```python
from build123d import *

# Parameters (mm, degrees)
SKETCH1_W           = 50.8
SKETCH1_H           = 38.1
SKETCH1_R           = 2.38125
BOSS_EXTRUDE1_DEPTH = 25.4
CUT_EXTRUDE1_DEPTH  = 58.410261207
FILLET1_R           = 6.35
SKETCH3_R           = 2.921
CUT_EXTRUDE2_DEPTH  = 25.4


with BuildPart() as part:
    # Sketch1 → Boss-Extrude1 (new body)
    with BuildSketch(Plane(origin=(0, 0, 0), x_dir=(1, 0, 0), z_dir=(0, 1, 0))):
        with Locations((-9.229006509, -1.483233189)):
            Rectangle(SKETCH1_W, SKETCH1_H)
        with Locations(Location((-28.279006509, 7.406766811, 0), (0, 0, 270))):
            Circle(SKETCH1_R, mode=Mode.SUBTRACT)
        with Locations(Location((-28.279006509, -1.483233189, 0), (0, 0, 270))):
            Circle(SKETCH1_R, mode=Mode.SUBTRACT)
        with Locations(Location((-28.279006509, -10.373233189, 0), (0, 0, 270))):
            Circle(SKETCH1_R, mode=Mode.SUBTRACT)
        with Locations(Location((9.820993491, -10.373233189, 0), (0, 0, 270))):
            Circle(SKETCH1_R, mode=Mode.SUBTRACT)
        with Locations(Location((9.820993491, -1.483233189, 0), (0, 0, 270))):
            Circle(SKETCH1_R, mode=Mode.SUBTRACT)
        with Locations(Location((9.820993491, 7.406766811, 0), (0, 0, 270))):
            Circle(SKETCH1_R, mode=Mode.SUBTRACT)
    extrude(amount=BOSS_EXTRUDE1_DEPTH)

    # Sketch2 → Cut-Extrude1 (cut, through all)
    with BuildSketch(Plane.XY.offset(20.533233189)):
        with BuildLine():
            Line((-21.929006509, 0), (3.470993491, 0))
            ThreePointArc((3.470993491, 0), (-9.229006509, 12.7), (-21.929006509, 0))
        make_face()
        Polygon((-25.739006509, 25.4), (7.280993491, 25.4), (16.170993491, 25.4), (16.170993491, 6.35), (3.470993491, 6.35), (3.470993491, 19.05), (-21.929006509, 19.05), (-21.929006509, 6.35), (-34.629006509, 6.35), (-34.629006509, 25.4), align=None)
    extrude(amount=-CUT_EXTRUDE1_DEPTH, mode=Mode.SUBTRACT)

    # Fillet1
    # the kernel refuses this fillet: 6.35 mm, written as the material it adds along each edge
    with BuildSketch(Plane(origin=(3.470993491, 6.35, 20.533233189), x_dir=(1, 0, 0), z_dir=(0, 0, -1))) as fillet1_piece_1_section:
        with BuildLine():
            CenterArc((FILLET1_R, -FILLET1_R), FILLET1_R, 90, 90)
            Line((0, -FILLET1_R), (0, 0))
            Line((0, 0), (FILLET1_R, 0))
        make_face()
    fillet1_piece_1 = extrude(amount=38.1, mode=Mode.PRIVATE)
    fillet1_piece_1 = fillet1_piece_1 - Plane(origin=(9.820993491, 7.811257132, -7.406766811), x_dir=(0, 0, 1), z_dir=(0, -1, 0)) * Cylinder(2.38125, 102, mode=Mode.PRIVATE)
    fillet1_piece_1 = fillet1_piece_1 - Plane(origin=(9.820993491, 7.811257132, 1.483233189), x_dir=(0, 0, 1), z_dir=(0, -1, 0)) * Cylinder(2.38125, 102, mode=Mode.PRIVATE)
    fillet1_piece_1 = fillet1_piece_1 - Plane(origin=(9.820993491, 7.811257132, 10.373233189), x_dir=(0, 0, 1), z_dir=(0, -1, 0)) * Cylinder(2.38125, 102, mode=Mode.PRIVATE)
    add(fillet1_piece_1)
    with BuildSketch(Plane(origin=(-21.929006509, 6.35, 20.533233189), x_dir=(0, 1, 0), z_dir=(0, 0, -1))) as fillet1_piece_2_section:
        with BuildLine():
            CenterArc((FILLET1_R, -FILLET1_R), FILLET1_R, 90, 90)
            Line((0, -FILLET1_R), (0, 0))
            Line((0, 0), (FILLET1_R, 0))
        make_face()
    fillet1_piece_2 = extrude(amount=38.1, mode=Mode.PRIVATE)
    fillet1_piece_2 = fillet1_piece_2 - Plane(origin=(-28.279006509, 7.811257363, -7.406766811), x_dir=(0, 0, 1), z_dir=(0, -1, 0)) * Cylinder(2.38125, 102, mode=Mode.PRIVATE)
    fillet1_piece_2 = fillet1_piece_2 - Plane(origin=(-28.279006509, 7.811257363, 1.483233189), x_dir=(0, 0, 1), z_dir=(0, -1, 0)) * Cylinder(2.38125, 102, mode=Mode.PRIVATE)
    fillet1_piece_2 = fillet1_piece_2 - Plane(origin=(-28.279006509, 7.811257363, 10.373233189), x_dir=(0, 0, 1), z_dir=(0, -1, 0)) * Cylinder(2.38125, 102, mode=Mode.PRIVATE)
    add(fillet1_piece_2)
    # the kernel refuses this fillet: 6.35 mm, written as the material it takes off along each edge
    with BuildSketch(Plane(origin=(3.470993491, 19.05, 36.408233189), x_dir=(0, -1, 0), z_dir=(0, 0, -1)), Plane(origin=(-21.929006509, 19.05, 36.408233189), x_dir=(1, 0, 0), z_dir=(0, 0, -1))) as fillet1_2_piece_1:
        with BuildLine():
            CenterArc((FILLET1_R, FILLET1_R), FILLET1_R, 180, 90)
            Line((0, FILLET1_R), (0, 0))
            Line((0, 0), (FILLET1_R, 0))
        make_face()
    extrude(amount=69.85, mode=Mode.SUBTRACT)

    # Sketch3 → Cut-Extrude2 (cut)
    with BuildSketch(Plane(origin=(0, 19.05, 0), x_dir=(1, 0, 0), z_dir=(0, 1, 0))):
        with Locations(Location((-9.229006509, -1.483233189, 0), (0, 0, 270))):
            Circle(SKETCH3_R)
        with Locations(Location((-9.229006509, 7.406766811, 0), (0, 0, 270))):
            Circle(SKETCH3_R)
        with Locations(Location((-9.229006509, -10.373233189, 0), (0, 0, 270))):
            Circle(SKETCH3_R)
    extrude(amount=-CUT_EXTRUDE2_DEPTH, mode=Mode.SUBTRACT)


solid = part.part
```
Geometry check sheet. Reference: the model listing, model coordinates, mm. A direction names the side the tool comes from. Round coordinates to 2 decimals unless told otherwise and drop trailing zeros. Loops run counter-clockwise (first coordinate to the right, second up) from the corner with the lowest first, then second, coordinate; pieces in that order, holes last. Notation, with made-up numbers: (45.5, -34.5) - (95.5, -34.5) arc R12 ccw to (95.5, -19.5) - close; hole circle Ø6 at (78.5, -15). An arc over 180 degrees is marked (long way). Use a Markdown table: item, result.
Q1. Cross-section at C-C on y = 16.5. Record the cut outline in (x, z).
Solutions:
| item | result |
|---|---|
| outline | (-20.67, -17.57) - (2.21, -17.57) - (2.21, 20.53) - (-20.67, 20.53) - close; hole circle Ø5.84 at (-9.23, -7.41); hole circle Ø5.84 at (-9.23, 1.48); hole circle Ø5.84 at (-9.23, 10.37) |
Q2. Cross-section at A-A on y = 7.5. Record the cut outline in (x, z), plus the area to 3 significant figures.
Solutions:
| item | result |
|---|---|
| outline | (-24.63, -17.57) - (-19.48, -17.57) - (-19.48, 20.53) - (-24.63, 20.53) - close; (1.02, -17.57) - (6.18, -17.57) - (6.18, 20.53) - (1.02, 20.53) - close |
| area | 393 mm2 |
Q3. Go/stop test with flat-tipped pins: P1, Ø6.5, axis at x = -9.23, z = -7.41, coming from the -Y side; P2, Ø9.5, axis at x = -9.23, z = 1.48, coming from the -Y side; P3, Ø9.5, axis at x = -9.23, z = 10.37, coming from the +Y side; P4, Ø1.9, axis at x = 13, z = -2, coming from the +Y side. Record where each tip stops, or that it passes through.
Solutions:
| item | result |
|---|---|
| P1 | stops at y = 12.28 |
| P2 | stops at y = 11.78 |
| P3 | stops at y = 19.05 |
| P4 | stops at y = 6.35 |
Q4. Access from +Z, -Z, +X, -X, +Y, -Y to the whole of each face (thin tool, end or side, straight path). Record for faces 4 (the cylindrical face through (-12.08, 15.75, 0.85)), 5 (the flat face through (-31, 6.35, 2)).
Solutions:
| item | result |
|---|---|
| face 4 | +Y, -Y |
| face 5 | +Z, -Z, -X, +Y |
Q5. Material ranges on line 1 (X direction, y = 5, z = 11); line 2 (X direction, y = 4.5, z = -9); line 3 (Z direction, x = -7.5, y = 13), recorded low to high.
Solutions:
| item | result |
|---|---|
| line 1 | x = -34.63 to -30.58, -25.98 to -20.9, 2.45 to 7.52, 12.12 to 16.17 |
| line 2 | x = -34.63 to -30.05, -26.51 to -21.11, 2.65 to 8.05, 11.59 to 16.17 |
| line 3 | z = -17.57 to -9.76, -5.05 to -0.87, 3.84 to 8.02, 12.73 to 20.53 |
Q6. Draft check along Z on faces 1 (the flat face through (13, 6.35, 2)), 2 (the cylindrical face through (-11.01, 15.75, -9.72)), 3 (the flat face through (-9, 14, 20.533)). Enter one of: released by +Z, released by -Z, zero draft, split by the parting line, or undercut.
Solutions:
| item | result |
|---|---|
| face 1 | zero draft |
| face 2 | undercut |
| face 3 | released by +Z |
Q7. Cross-section at D-D on x = -25. Record the cut outline in (y, z), plus the area to 3 significant figures.
Solutions:
| item | result |
|---|---|
| outline | (0, -17.57) - (7.26, -17.57) - (7.26, 20.53) - (0, 20.53) - close |
| area | 277 mm2 |
Q8. Cross-section at B-B on z = 5.5. Record the cut outline in (x, y), plus the area to 3 significant figures.
Solutions:
| item | result |
|---|---|
| outline | (-34.63, 0) - (-21.93, 0) arc R12.7 cw to (3.47, 0) - (16.17, 0) - (16.17, 6.35) - (9.82, 6.35) arc R6.35 cw to (3.47, 12.7) arc R6.35 ccw to (-2.88, 19.05) - (-15.58, 19.05) arc R6.35 ccw to (-21.93, 12.7) arc R6.35 cw to (-28.28, 6.35) - (-34.63, 6.35) - close |
| area | 392 mm2 |
